from build123d import *

# Parameters (mm, degrees)
F1_DEPTH = 8
F2_SIZE  = 0.5
F3_SIZE  = 0.8
F4_R     = 1


with BuildPart() as f1:
    # F0 (on Front) → F1 (new body)
    with BuildSketch(Plane.XZ):
        with BuildLine():
            Line((0, 6.6), (0, 0))
            Line((0, 0), (-1.3, 0))
            Line((-1.3, 0), (-1.3, -1.5))
            Line((-1.3, -1.5), (0.8, -1.5))
            Line((0.8, -1.5), (0.8, 0))
            Line((0.8, 0), (0.8, 7.4))
            Line((0.8, 7.4), (-3.5, 7.4))
            Line((-3.5, 7.4), (-4.375, 7.4))
            Line((-4.375, 7.4), (-5.805823, 4.768717))
            ThreePointArc((-5.805823, 4.768717), (-6.047673, 3.794818), (-5.690622, 2.857009))
            Line((-5.690622, 2.857009), (-4.375, 1.187434))
            Line((-4.375, 1.187434), (-3.5, 1.187434))
            Line((-3.5, 1.187434), (-3.5, 3.018717))
            Line((-3.5, 3.018717), (-4.375, 3.018717))
            ThreePointArc((-4.375, 3.018717), (-5.25, 3.893717), (-4.375, 4.768717))
            Line((-4.375, 4.768717), (-3.5, 4.768717))
            Line((-3.5, 4.768717), (-3.5, 6.6))
            Line((-3.5, 6.6), (0, 6.6))
        make_face()
    extrude(amount=F1_DEPTH)

    # F2
    f2_edges = [f1.edges().sort_by_distance(p)[0] for p in [
        (0, -4, 0),
    ]]
    chamfer(f2_edges, length=F2_SIZE)

    # F3
    f3_edges = [f1.edges().sort_by_distance(p)[0] for p in [
        (-1.3, -4, -1.5),
    ]]
    chamfer(f3_edges, length=F3_SIZE)

    # F4
    f4_edges = [f1.edges().sort_by_distance(p)[0] for p in [
        (-4.375, -4, 1.187434),
        (-4.375, -4, 7.4),
    ]]
    fillet(f4_edges, radius=F4_R)


solid = f1.part
Could you check a few things on this model? Use its own coordinates, in mm. A direction names the side the tool comes from. Give positions to 0.01 mm unless a question says otherwise; leave off trailing zeros. Loops run counter-clockwise (first coordinate to the right, second up) from the corner with the lowest first, then second, coordinate; pieces in that order, holes last. Notation, with made-up numbers: (-13.75, 6) -> (13.25, 6) arc R24 ccw to (13.25, 36) -> close; hole circle Ø10 at (-12, -28). An arc over 180 degrees is marked (long way). Answer as CSV lines item,"result". Start each with the question number.
(1) If we section it at A-A on x = -0.25: Write out the boundary of the cut face in (y, z).
(2) I'm going to push flat-ended pins straight in: pin 1 Ø1 at (x, y) = (-2.5, -5) entering from -Z; pin 2 Ø0.7 at (x, y) = (-4, -4) entering from -Z; pin 3 Ø1 at (x, y) = (-1.5, -3) entering from -Z. Where does each tip first touch, or does it pass through?
(3) If we section it at B-B on z = 3.5: Write out the boundary of the cut face in (x, y).
(4) We'd pull the mould along X, two halves only. Please class faces 4 (the flat face through (-5.19, -3.94, 2.22)), 5 (the flat face through (-3.5, -4, 2)), 6 (the flat face through (-1, -4, 7.4)): released by +X, released by -X, zero draft, split by the parting line, or undercut.
(5) Which directions (+Z, -Z, +X, -X, +Y, -Y) give clear straight access to the entire face, cutting with the end or side of a thin tool? Please do faces 1 (the flat face through (-5.224, -3.944, 5.838)), 2 (the flat face through (-2, -4, 6.6)), 3 (the flat face through (-3.5, -4, 6)).
(6) I need wall thicknesses on probe 1 along Z at (x, y) = (-1.75, -0.5); probe 2 along X at (y, z) = (-6, 2.5); probe 3 along Z at (x, y) = (-3.75, -2.5). Which ranges of each line are inside material? Lowest first, please.
Computed:
1,outline,"(-8, -1.5) -> (0, -1.5) -> (0, 0.25) -> (-8, 0.25) -> close; (-8, 6.6) -> (0, 6.6) -> (0, 7.4) -> (-8, 7.4) -> close"
2,pin 1,"stops at z = 6.6"
2,pin 2,"stops at z = 1.19"
2,pin 3,"stops at z = -1"
3,outline,"(-6, -8) -> (-5.16, -8) -> (-5.16, 0) -> (-6, 0) -> close; (0, -8) -> (0.8, -8) -> (0.8, 0) -> (0, 0) -> close"
4,face 4,"released by -X"
4,face 5,"undercut"
4,face 6,"zero draft"
5,face 1,"+Z, -X, +Y, -Y"
5,face 2,"+Y, -Y"
5,face 3,"-Z, +Y, -Y"
6,probe 1,"z = 6.6 to 7.4"
6,probe 2,"x = -5.41 to -3.5, 0 to 0.8"
6,probe 3,"z = 1.19 to 3.02, 4.77 to 7.4"
